Design review of the part built by this model. Coordinates are the model's own, in mm. Coordinates: 2 decimals unless noted, no trailing zeros. Loops run counter-clockwise (first coordinate to the right, second up) from the corner with the lowest first, then second, coordinate; pieces in that order, holes last. Notation, with made-up numbers: (33.5, 31) - (43.5, 31) arc R11 cw to (43.5, 52) - close; hole circle Ø6 at (12, 4.25). An arc over 180 degrees is marked (long way). One line per question, with ' | ' between items.
from build123d import *

# Parameters (mm, degrees)
BOSS_EXTRUDE1_DEPTH = 3.175
SKETCH2_R           = 1.5875
CUT_EXTRUDE1_DEPTH  = 3.175
BOSS_EXTRUDE2_DEPTH = 3.175
CUT_EXTRUDE2_DEPTH  = 3.175
CUT_EXTRUDE3_DEPTH  = 10.16
LPATTERN1_COUNT     = 4
LPATTERN1_PITCH     = 25.4
SKETCH6_W           = 12.7
SKETCH6_H           = 3.048
CUT_EXTRUDE4_DEPTH  = 5.08
LPATTERN2_COUNT     = 3
LPATTERN2_PITCH     = 31.75
SKETCH7_R           = 1.5875
CUT_EXTRUDE5_DEPTH  = 19.05


with BuildPart() as part:
    # Sketch1 → Boss-Extrude1 (new body)
    with BuildSketch(Plane.XY):
        Polygon((0, 0), (-177.8, 0), (-232.7656, 382.27), (-80.3656, 382.27), align=None)
    extrude(amount=BOSS_EXTRUDE1_DEPTH)

    # Sketch2 → Cut-Extrude1 (cut)
    with BuildSketch(Plane.XY.offset(3.175)):
        with Locations((-127, 127)):
            Circle(SKETCH2_R)
        with Locations((-181.95798, 335.788)):
            Circle(SKETCH2_R)
    extrude(amount=-CUT_EXTRUDE1_DEPTH, mode=Mode.SUBTRACT)

    # Sketch3 → Boss-Extrude2 (add)
    with BuildSketch(Plane.XY.offset(3.175)):
        Polygon((-63.5, 82.55), (63.5, 104.94352655), (63.5, 181.14352655), (-63.5, 181.14352655), align=None)
    extrude(amount=-BOSS_EXTRUDE2_DEPTH)

    # Sketch4 → Cut-Extrude2 (cut)
    with BuildSketch(Plane.XY.offset(3.175)):
        Polygon((-57.15, 104.14), (-44.642941537, 106.345331856), (-45.194274501, 109.472096472), (-57.701332964, 107.266764616), align=None)
        Polygon((-19.62882461, 110.755995569), (-7.121766147, 112.961327425), (-7.673099111, 116.088092041), (-20.180157574, 113.882760185), align=None)
    extrude(amount=-CUT_EXTRUDE2_DEPTH, mode=Mode.SUBTRACT)

    # Sketch5 → Cut-Extrude3 (cut)
    with BuildSketch(Plane.XY.offset(3.175)):
        Polygon((-148.01334563, 206.830707159), (-144.780523225, 194.549059903), (-143.245317319, 194.953162704), (-146.478139723, 207.234809959), align=None)
        Polygon((-146.315729132, 194.144957103), (-144.780523225, 194.549059903), (-148.01334563, 206.830707159), (-149.548551537, 206.426604358), align=None)
    cut_extrude3 = extrude(amount=-CUT_EXTRUDE3_DEPTH, mode=Mode.SUBTRACT)

    # LPattern1: Cut-Extrude3 ×4
    with Locations(*[Vector(-0.254552945, 0.967058839, 0) * (i * LPATTERN1_PITCH) for i in range(1, LPATTERN1_COUNT)]):
        add(cut_extrude3, mode=Mode.SUBTRACT)

    # Sketch6 → Cut-Extrude4 (cut)
    with BuildSketch(Plane.XY.offset(3.175)):
        with Locations((-158.75, 51.181)):
            Rectangle(SKETCH6_W, SKETCH6_H)
    cut_extrude4 = extrude(amount=-CUT_EXTRUDE4_DEPTH, mode=Mode.SUBTRACT)

    # LPattern2: Cut-Extrude4 ×3
    with Locations(*[(i * LPATTERN2_PITCH, 0, 0) for i in range(1, LPATTERN2_COUNT)]):
        add(cut_extrude4, mode=Mode.SUBTRACT)

    # Sketch7 → Cut-Extrude5 (cut)
    with BuildSketch(Plane.XY.offset(3.175)):
        with Locations((-152.4, 29.337)):
            Circle(SKETCH7_R)
        with Locations((-101.6, 29.337)):
            Circle(SKETCH7_R)
    extrude(amount=-CUT_EXTRUDE5_DEPTH, mode=Mode.SUBTRACT)


solid = part.part
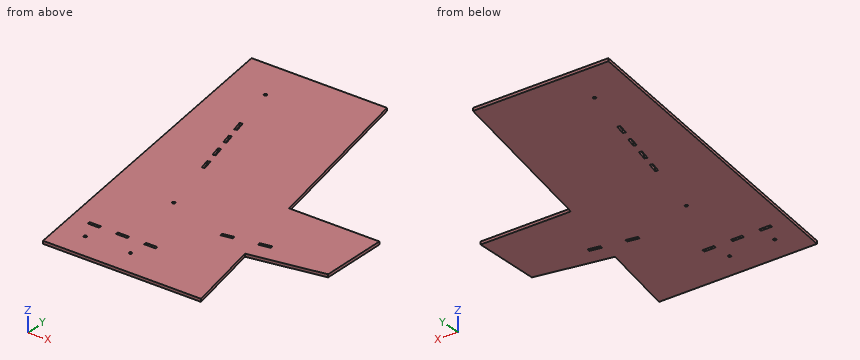
Q1. Take a section at B-B (y = 346.5). Give the boundary of the cut face in (x, z) (3 decimals), plus the area to 3 significant figures.
Returned:
outline: (-227.622, 0) - (-72.846, 0) - (-72.846, 3.175) - (-227.622, 3.175) - close | area: 491 mm²
Q2. For pin 1 (2.5 mm diameter, centred on x = -127, y = 127, fed in from +Z); pin 2 (1.5 mm diameter, centred on y = 52, z = 1.5, fed in from +X); pin 3 (1 mm diameter, centred on y = 140.5, z = 2.5, fed in from -X); pin 4 (1 mm diameter, centred on y = 82, z = 3, fed in from -X), all flat-tipped, find the tip position at first contact; note any pin that passes through.
Returned:
pin 1: passes through | pin 2: stops at x = -10.77 | pin 3: stops at x = -198.07 | pin 4: stops at x = -189.66
Q3. To check wall thickness, follow line 1 along Y through (x, z) = (-127, 1.9) (1 decimal); line 2 along X through (y, z) = (126, 0.25); line 3 along Y through (x, z) = (-24.5, 0.7). State the ranges of each line that lie inside material, in increasing order.
Returned:
line 1: y = 0 to 49.7, 52.7 to 125.4, 128.6 to 382.3 | line 2: x = -195.92 to -128.23, -125.77 to 63.5 | line 3: y = 0 to 181.14
Q4. Take a section at A-A (z = 1.25). State how many separate pieces and enclosed holes the cut face has, plus the area to 3 significant figures.
Returned:
separate pieces: 1 | enclosed holes: 13 | area: 70,500 mm²
Q5. Take a section at C-C (y = 148.5). Give the boundary of the cut face in (x, z) (3 decimals), plus the area to 3 significant figures.
Returned:
outline: (-199.152, 0) - (63.5, 0) - (63.5, 3.175) - (-199.152, 3.175) - close | area: 834 mm²
